from build123d import *

# Parameters (mm, degrees)
SKETCH_1_R      = 9
EXTRUDE_1_DEPTH = 48
SKETCH_2_R      = 12
EXTRUDE_2_DEPTH = 4
FILLET_1_R      = 0.5
FILLET_2_R      = 0.5


with BuildPart() as part:
    # 草图1 → 凸台-拉伸1 (new body)
    with BuildSketch(Plane(origin=(0, 0, 0), x_dir=(0, 0, -1), z_dir=(1, 0, 0))):
        Circle(SKETCH_1_R)
    extrude(amount=-EXTRUDE_1_DEPTH)

    # 草图2 → 凸台-拉伸2 (add)
    with BuildSketch(Plane(origin=(0, 0, 0), x_dir=(0, 0, -1), z_dir=(1, 0, 0))):
        Circle(SKETCH_2_R)
    extrude(amount=EXTRUDE_2_DEPTH)

    # 圆角1
    fillet_1_edges = [part.edges().sort_by_distance(p)[0] for p in [
        (4, 0, 12),
    ]]
    fillet(fillet_1_edges, radius=FILLET_1_R)

    # 圆角2
    fillet_2_edges = [part.edges().sort_by_distance(p)[0] for p in [
        (-48, 0, 9),
    ]]
    fillet(fillet_2_edges, radius=FILLET_2_R)


solid = part.part
Design review of the part built by this model. Coordinates are the model's own, in mm. A direction names the side the tool comes from. Round coordinates to 2 decimals unless told otherwise and drop trailing zeros. Loops run counter-clockwise (first coordinate to the right, second up) from the corner with the lowest first, then second, coordinate; pieces in that order, holes last. Notation, with made-up numbers: (56, 67) - (103, 67) arc R24 cw to (103, 102) - close; hole circle Ø6 at (43.5, 42). An arc over 180 degrees is marked (long way). One line per question, with ' | ' between items.
1. For faces 1 (the face through (-23.418, 8.923, 1.172)), 2 (the face through (-48, 0, 0)), list the 3-axis set-ups (+Z, -Z, +X, -X, +Y, -Y) from which the entire face can be reached by the end or side of a thin tool; tool diameter is ignored.
Results are:
face 1: -X | face 2: +Z, -Z, -X, +Y, -Y
2. We need section C-C, the plane x = -39. State the section outline as (y, z) points, and give its area (3 significant figures).
Results are:
outline: circle Ø18 at (0, 0) | area: 254 mm²
3. Clearance check with flat-ended pins moving along their axes: P1, Ø10, axis at x = -30, z = 3, coming from the -Y side; P2, Ø1, axis at x = -10, z = 7, coming from the -Y side; P3, Ø1, axis at x = -34, z = -2, coming from the +Y side. State where each tip first meets the part, or that it passes through.
Results are:
P1: stops at y = -9 | P2: stops at y = -6.22 | P3: stops at y = 8.87
4. We need section A-A, the plane y = 0. State the section outline as (x, z) points, and give its area (3 significant figures).
Results are:
outline: (-48, -8.5) arc R0.5 ccw to (-47.5, -9) - (0, -9) - (0, -12) - (3.5, -12) arc R0.5 ccw to (4, -11.5) - (4, 11.5) arc R0.5 ccw to (3.5, 12) - (0, 12) - (0, 9) - (-47.5, 9) arc R0.5 ccw to (-48, 8.5) - close | area: 960 mm²
5. For L1, parallel to X at y = -10.5, z = -1.25; L2, parallel to Z at x = -0.5, y = 0.25; L3, parallel to X at y = 8.75, z = -1.5, list the stretches that pass through material, from the lowest coordinate up. Write a range as [from, to].
Results are:
L1: x = [0, 4] | L2: z = [-9, 9] | L3: x = [-47.83, 4]
